The listing builds one solid part. Answer for the finished solid, in the listing's coordinates (mm). Face numbers are marked on the shaded views. A direction names the side the tool comes from. Round coordinates to 2 decimals unless told otherwise and drop trailing zeros. Write each loop counter-clockwise with the first axis right and the second up, starting at its lowest first coordinate (ties: lowest second). Pieces come first, ordered by that corner, then holes.
(1) The mould has two halves that part along Z. Classify the marked faces 1, 2 and 3: +Z half, -Z half, draft (parallel to the pull), parting line (faces both ways), or undercut.
(2) A cutting plane is placed at A-A, the plane x = 23. Give the vertices of the cut face in (y, z).
(3) Find the intervals of material crossed by probe 1 along Y at (x, z) = (56, 55); probe 2 along Z at (x, y) = (41, 62.5); probe 3 along Y at (x, z) = (26, 32), in increasing order.
(4) Each of these flat-tipped pins is pushed along its axis until it touches: pin 1 Ø10 at (y, z) = (11, 94) entering from +X; pin 2 Ø1.5 at (y, z) = (17, 13.5) entering from +X; pin 3 Ø19 at (x, z) = (48.5, 52.5) entering from -Y; pin 4 Ø1.5 at (x, z) = (10.5, 50) entering from -Y. Where does it stop, or does it pass through?
(5) For the marked faces 4, 5 and 6, determine the directions among +Z, -Z, +X, -X, +Y, -Y from which every point of the face is accessible in a straight line to the end or side of a thin tool.
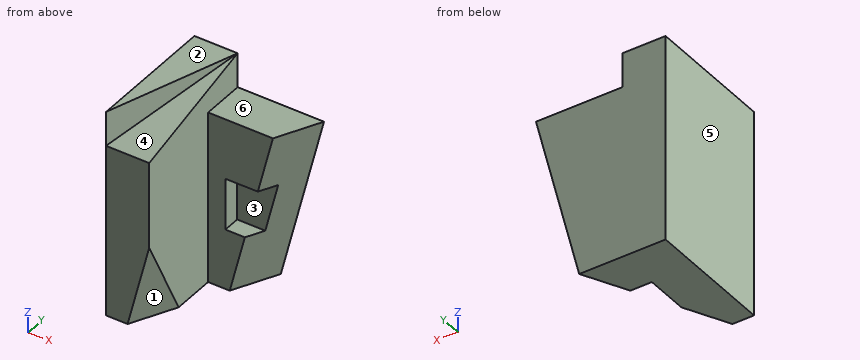
from build123d import *

# Parameters (mm, degrees)
F0_W      = 25
F0_H      = 75
F1_DEPTH  = 120
F6_W      = 25
F6_H      = 20
F12_W     = 35
F12_H     = 30
F13_DEPTH = 60


with BuildPart() as f1:
    # F0 (on Top) → F1 (new body)
    with BuildSketch(Plane.XY):
        with Locations((12.5, 37.5)):
            Rectangle(F0_W, F0_H)
    extrude(amount=F1_DEPTH)

    # F2 (on Top) → F5 section 0
    with BuildSketch(Plane.XY):
        Polygon((50, 75), (25, 75), (25, 50), (37.5, 50), align=None)
    # F4 (on offset) → F5 section 1
    with BuildSketch(Plane.XY.offset(100)):
        Polygon((75, 75), (25, 75), (25, 50), (62.5, 50), align=None)
    loft()

    # F6 (on face) → F8 section 0
    with BuildSketch(Plane.XZ, mode=Mode.PRIVATE) as f8_s0:
        with Locations((12.5, 110)):
            Rectangle(F6_W, F6_H)
    loft([f8_s0.sketch, Vertex(25, 75, 120)], mode=Mode.SUBTRACT)

    # F9 (on face) → F11 section 0
    with BuildSketch(Plane(origin=(0, 0, 0), x_dir=(1, 0, 0), z_dir=(0, 0, -1)), mode=Mode.PRIVATE) as f11_s0:
        Polygon((25, 0), (12.5, 0), (25, -25), align=None)
    loft([f11_s0.sketch, Vertex(25, 0, 50)], mode=Mode.SUBTRACT)

    # F12 (on face) → F13 (cut)
    with BuildSketch(Plane.XZ):
        with Locations((52.5, 50)):
            Rectangle(F12_W, F12_H)
    extrude(amount=-F13_DEPTH, mode=Mode.SUBTRACT)


solid = f1.part
Solutions:
1. face 1: -Z half
1. face 2: +Z half
1. face 3: undercut
2. outline: (0, 42) - (21, 0) - (75, 0) - (75, 120) - (69, 120) - (69, 118.4) - (0, 100) - close
3. probe 1: y = 60 to 75
3. probe 2: z = 0 to 100
3. probe 3: y = 50 to 75
4. pin 1: stops at x = 25
4. pin 2: stops at x = 24.79
4. pin 3: stops at y = 60
4. pin 4: stops at y = 0
5. face 4: +Z, +X, -Y
5. face 5: +Z, -Z, -X, +Y, -Y
5. face 6: +Z, +X, +Y, -Y
